Answer from the drawing. Dimensions are ordinates in mm from the lowest x, y and z of the part. A direction names the side the tool comes from. Coordinates: 2 decimals unless noted, no trailing zeros. Order: outer loops, then holes, each group sorted by start corner. A loop starts at its lowest first (then second) coordinate and runs counter-clockwise, first axis right, second up. Notation, with made-up numbers: (22.25, -15) - (63.25, -15) arc R24 ccw to (63.25, 18) - close; hole circle Ø6 at (51.5, 33.25). An arc over 180 degrees is marked (long way). Use a Markdown table: item, result. Add a question column.
Item 1: Flat-ended cylindrical pins translate along their axes: P1, Ø5, axis at x = 21.5, z = 16.5, coming from the +Y side; P2, Ø6, axis at x = 23.5, z = 6.5, coming from the -Y side; P3, Ø1.5, axis at x = 13, y = 14.5, coming from the +Z side. Find the tip coordinate at first contact, or state that the pin passes through.
Item 2: The part is cut by section A-A, the plane y = 9.25. Give the vertices of the cut face in (x, z), then the cut area to 3 significant figures.
Item 3: The part is cut by section C-C, the plane x = 26.5. Give the vertices of the cut face in (y, z), then the cut area to 3 significant figures.
Item 4: The part is cut by section D-D, the plane x = 9.5. Give the vertices of the cut face in (y, z), then the cut area to 3 significant figures.
Item 5: Find the intervals of material crossed by line 1 along Y through (x, z) = (16.5, 9.25); line 2 along X through (y, z) = (4.5, 16); line 3 along Y through (x, z) = (1, 11), in increasing order.
Item 6: The mould has two halves that part along Z. Classify the marked faces 3, 4 and 5: released by +Z, released by -Z, zero draft, split by the parting line, or undercut.
Item 7: For the marked faces 1 and 2, determine the directions among +Z, -Z, +X, -X, +Y, -Y from which every point of the face is accessible in a straight line to the end or side of a thin tool.
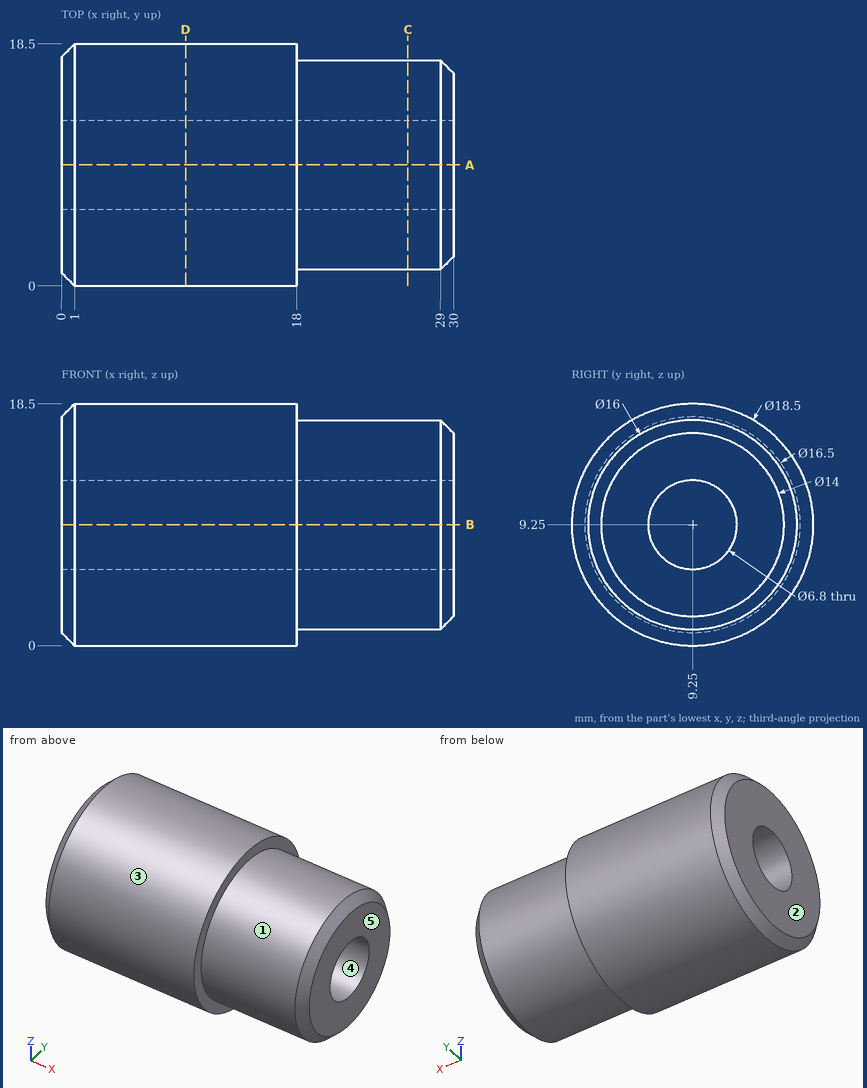
Solution:
| question | item | result |
|---|---|---|
| 1 | P1 | stops at y = 15.69 |
| 1 | P2 | stops at y = 1.25 |
| 1 | P3 | stops at z = 17.33 |
| 2 | outline | (0, 1) - (1, 0) - (18, 0) - (18, 1.25) - (29, 1.25) - (30, 2.25) - (30, 5.85) - (0, 5.85) - close; (0, 12.65) - (30, 12.65) - (30, 16.25) - (29, 17.25) - (18, 17.25) - (18, 18.5) - (1, 18.5) - (0, 17.5) - close |
| 2 | area | 319 mm2 |
| 3 | outline | circle Ø16 at (9.25, 9.25); hole circle Ø6.8 at (9.25, 9.25) |
| 3 | area | 165 mm2 |
| 4 | outline | circle Ø18.5 at (9.25, 9.25); hole circle Ø6.8 at (9.25, 9.25) |
| 4 | area | 232 mm2 |
| 5 | line 1 | y = 0 to 5.85, 12.65 to 18.5 |
| 5 | line 2 | x = 0 to 18 |
| 5 | line 3 | y = 0.17 to 6.33, 12.17 to 18.33 |
| 6 | face 3 | split by the parting line |
| 6 | face 4 | undercut |
| 6 | face 5 | zero draft |
| 7 | face 1 | +X |
| 7 | face 2 | +Z, -Z, -X, +Y, -Y |
